Autodesk Inventor part; units mm, degrees
ref_plane "YZ Plane" through (0, 0, 0) normal (1, 0, 0) x (0, 1, 0)
ref_plane "XZ Plane" through (0, 0, 0) normal (0, 1, 0) x (-1, 0, 0)
ref_plane "XY Plane" through (0, 0, 0) normal (0, 0, 1) x (1, 0, 0)
sketch "Sketch1" plane through (0, 0, 0) normal (0, 0, 1) x (1, 0, 0)
  circle A0 centre (0, 0) radius 7
  arc A1 (-3.096, -4.5458) -> (5.2116, 1.7576) centre (0, 0) ccw
  point P0 (0, 0)
  dimension "d0" = 14
extrude "Extrusion1" add sketch "Sketch1" along normal blind 10.5
sketch "Sketch2" plane through (0, 0, 10.5) normal (0, 0, 1) x (1, 0, 0)
  circle A0 centre (0, 0) radius 7
  line L0 (7, 0) -> (4.5, 0)
  circle A1 centre (4.5, 0) radius 2.125
  point P0 (0, 0)
  dimension "d3" = 2.5
  dimension "d4" = 4.25
extrude "Extrusion2" cut sketch "Sketch2" against normal blind 5 contours A1
sketch "Sketch3" plane through (0, 0, 0) normal (0, 0, -1) x (-1, 0, 0)
  circle A0 centre (0, 0) radius 5
  circle A1 centre (0, 0) radius 7
  circle A2 centre (0, 0) radius 6
  point P0 (0, 0)
  dimension "d7" = 12
extrude "Extrusion3" add sketch "Sketch3" along normal blind 3 contours A0 | A2
properties part number "RotationDisk"
Input: part model. Units: mm. Frame: model coordinates. A direction names the side the tool comes from. Coordinates: 2 decimals unless noted, no trailing zeros. Loops run counter-clockwise (first coordinate to the right, second up) from the corner with the lowest first, then second, coordinate; pieces in that order, holes last. Notation, with made-up numbers: (60, 5) -> (102, 5) arc R7 cw to (102, 10) -> close; hole circle Ø6 at (60.5, 60.5). An arc over 180 degrees is marked (long way). One line per item, written item: value.
(1) Cut plane A-A (x = 0). Output: boundary loops of the cut face in (y, z), then the cut area to 3 significant figures.
Answer below:
outline: (-7, 0) -> (-6, 0) -> (-6, -3) -> (6, -3) -> (6, 0) -> (7, 0) -> (7, 10.5) -> (-7, 10.5) -> close
area: 183 mm2
(2) Set-up query: faces 4 (the face through (2.377, 0.093, 8.035)), 5 (the face through (6, 2, 0)), 6 (the face through (0, 0, 10.5)). Return all of +Z, -Z, +X, -X, +Y, -Y with unobstructed straight access to the full face (end or side cutting, diameter ignored); none if empty.
Answer below:
face 4: +Z
face 5: -Z
face 6: +Z, +X, -X, +Y, -Y
(3) Pin query (flat end, axial travel): pin 1 Ø1 at (x, z) = (1.5, 4.5) entering from +Y; pin 2 Ø3 at (y, z) = (3, 6) entering from -X; pin 3 Ø3 at (y, z) = (-4.5, 6.5) entering from +X. Return the tip coordinate at first contact, or that it passes through.
Answer below:
pin 1: stops at y = 6.93
pin 2: stops at x = -6.84
pin 3: stops at x = 6.32
(4) Ray query, line 1 along Y through (x, z) = (-0.25, -0.5); line 2 along Y through (x, z) = (4.5, 8.7) (3 decimals); line 3 along Z through (x, y) = (4.5, -4.25). Return the intervals inside material, ascending.
Answer below:
line 1: y = -5.99 to 5.99
line 2: y = -5.362 to -2.125, 2.125 to 5.362
line 3: z = 0 to 10.5
(5) Draft query along Y for faces 1 (the face through (0, 0, -3)), 2 (the face through (6.466, 2.681, 5.176)), 3 (the face through (4, 0, 5.5)). Return one class per face: pulls with the +Y half, pulls with the -Y half, needs draft (parallel to the pull), parting line crosses it, or undercut.
Answer below:
face 1: needs draft
face 2: parting line crosses it
face 3: undercut
(6) Cut plane C-C (z = 4.5). Output: boundary loops of the cut face in (x, y), then the cut area to 3 significant figures.
Answer below:
outline: circle Ø14 at (0, 0)
area: 154 mm2
(7) Cut plane B-B (y = 0). Output: boundary loops of the cut face in (x, z) (3 decimals).
Answer below:
outline: (-7, 0) -> (-6, 0) -> (-6, -3) -> (6, -3) -> (6, 0) -> (7, 0) -> (7, 10.5) -> (6.625, 10.5) -> (6.625, 5.5) -> (2.375, 5.5) -> (2.375, 10.5) -> (-7, 10.5) -> close
(8) Cut plane D-D (y = 5.25). Output: boundary loops of the cut face in (x, z).
Answer below:
outline: (-4.63, 0) -> (-2.9, 0) -> (-2.9, -3) -> (2.9, -3) -> (2.9, 0) -> (4.63, 0) -> (4.63, 10.5) -> (-4.63, 10.5) -> close
